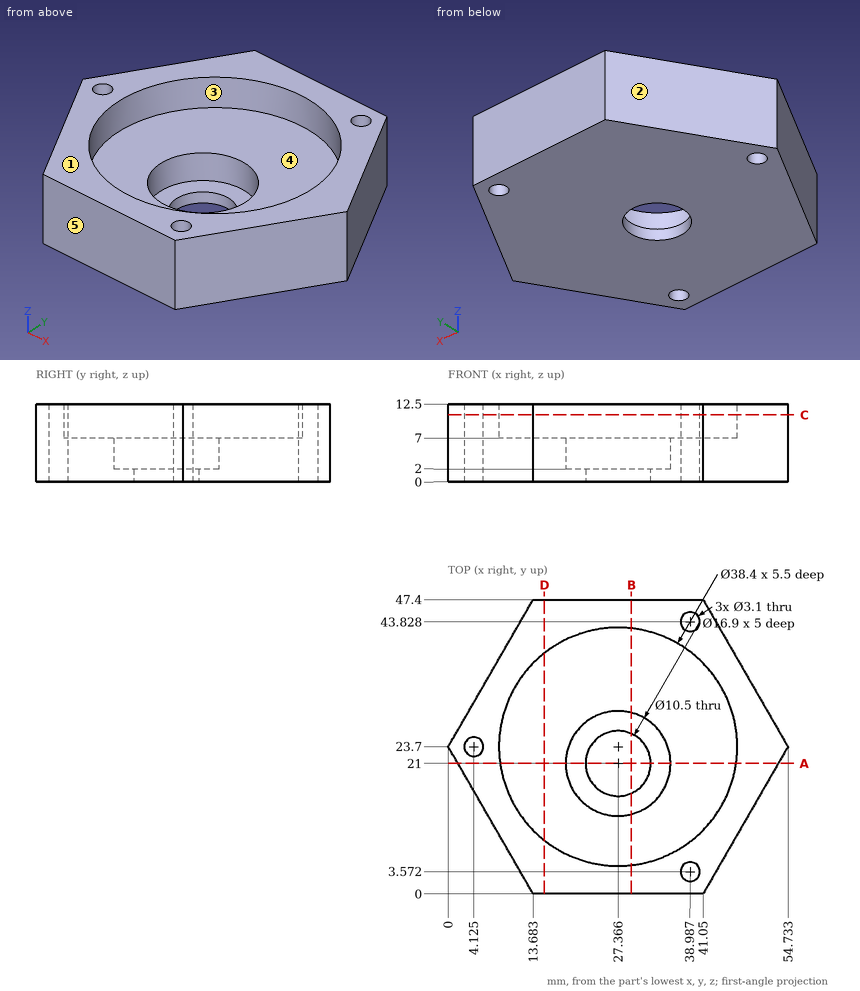
Study the drawing (mm; zero at the part's minimum x, y, z) and answer. A direction names the side the tool comes from. Coordinates: 2 decimals unless noted, no trailing zeros. Write each loop counter-clockwise with the first axis right and the second up, starting at its lowest first coordinate (ties: lowest second). Pieces come first, ordered by that corner, then holes.
Q1. Find the intervals of material crossed by line 1 along X through (y, z) = (24, 5) (1 decimal); line 2 along Z through (x, y) = (33, 42); line 3 along X through (y, z) = (33.5, 9) (1 decimal), in increasing order.
Returned:
line 1: x = 0.2 to 2.6, 5.6 to 19.5, 35.3 to 54.6
line 2: z = 0 to 7
line 3: x = 5.7 to 10.9, 43.9 to 49.1
Q2. Which of the six approach directions +Z, -Z, +X, -X, +Y, -Y give full straight-line access (tool end or side, diameter ignored) to the marked faces 4 and 5?
Returned:
face 4: +Z
face 5: +Z, -Z, +X, -X, -Y
Q3. Given P1, Ø1, axis at x = 44.5, z = 6.5, coming from the -Y side; P2, Ø3, axis at y = 6, z = 7, coming from the +X side; P3, Ø5, axis at x = 24.5, y = 24.5, coming from the +Z side, each flat-ended and moving along its own axis, determine where each tip first touches the part or whether it passes through.
Returned:
P1: stops at y = 5.11
P2: stops at x = 45.38
P3: stops at z = 2
Q4. Section D-D, the plane x = 15.5 is taken. Write down the section's boundary in (y, z).
Returned:
outline: (0, 0) - (47.4, 0) - (47.4, 12.5) - (38.79, 12.5) - (38.79, 7) - (8.61, 7) - (8.61, 12.5) - (0, 12.5) - close
Q5. The mould has two halves that part along X. Classify the marked faces 1, 2 and 3: released by +X, released by -X, zero draft, split by the parting line, or undercut.
Returned:
face 1: zero draft
face 2: released by -X
face 3: undercut
Q6. Section B-B, the plane x = 29.5 is taken. Write down the section's boundary in (y, z).
Returned:
outline: (0, 0) - (16.2, 0) - (16.2, 2) - (12.82, 2) - (12.82, 7) - (4.62, 7) - (4.62, 12.5) - (0, 12.5) - close; (25.8, 0) - (47.4, 0) - (47.4, 12.5) - (42.78, 12.5) - (42.78, 7) - (29.18, 7) - (29.18, 2) - (25.8, 2) - close
Q7. Section A-A, the plane y = 21 is taken. Write down the section's boundary in (x, z) (1 decimal).
Returned:
outline: (1.6, 0) - (22.1, 0) - (22.1, 2) - (18.9, 2) - (18.9, 7) - (8.4, 7) - (8.4, 12.5) - (1.6, 12.5) - close; (32.6, 0) - (53.2, 0) - (53.2, 12.5) - (46.4, 12.5) - (46.4, 7) - (35.8, 7) - (35.8, 2) - (32.6, 2) - close
Q8. Section C-C, the plane z = 10.75 is taken. Give the number of separate pieces and of enclosed holes in the cut face, then the cut area to 3 significant figures.
Returned:
separate pieces: 1
enclosed holes: 4
area: 765 mm2
